from build123d import *

# Parameters (mm, degrees)
SKETCH1_R           = 2.625
BOSS_EXTRUDE1_DEPTH = 6


with BuildPart() as part:
    # Sketch1 → Boss-Extrude1 (new body)
    with BuildSketch(Plane(origin=(0, 0, 0), x_dir=(1, 0, 0), z_dir=(0, 1, 0))):
        with BuildLine():
            Line((-7, 10), (7, 10))
            ThreePointArc((7, 10), (7.707106781, 9.707106781), (8, 9))
            Line((8, 9), (8, -9))
            ThreePointArc((8, -9), (7.707106781, -9.707106781), (7, -10))
            Line((7, -10), (-7, -10))
            ThreePointArc((-7, -10), (-7.707106781, -9.707106781), (-8, -9))
            Line((-8, -9), (-8, 9))
            ThreePointArc((-8, 9), (-7.707106781, 9.707106781), (-7, 10))
        make_face()
        Circle(SKETCH1_R, mode=Mode.SUBTRACT)
    extrude(amount=BOSS_EXTRUDE1_DEPTH)


solid = part.part
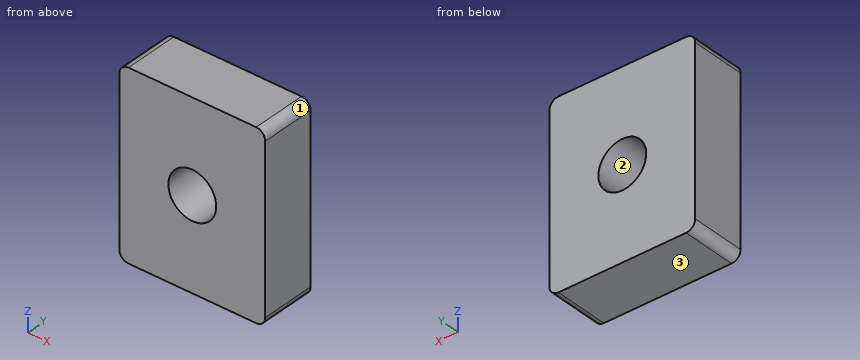
Verification items for the finished model (mm, model axes). Face numbers are marked on the shaded views. Coordinates: 2 decimals unless noted, no trailing zeros. Order: outer loops, then holes, each group sorted by start corner. A loop starts at its lowest first (then second) coordinate and runs counter-clockwise, first axis right, second up. Notation, with made-up numbers: M -15,49.5 L 41,49.5 A16 ccw 41,77.5 Z; hole C 2.25,34 d3. An arc over 180 degrees is marked long. One line per item, written item: value. Start each with the question number.
Item 1: Sectioned sample at C-C on x = 0. Record the cut outline in (y, z) (3 decimals).
Item 2: Thickness scan on probe 1 along X at (y, z) = (4.25, 0) (3 decimals); probe 2 along Z at (x, y) = (0, 3.5) (3 decimals); probe 3 along X at (y, z) = (0.8, 2). Record the ranges inside material, lowest first.
Item 3: Sectioned sample at B-B on y = 3.9. Record the cut outline in (x, z) (3 decimals), then the cut area to 3 significant figures.
Item 4: Sectioned sample at A-A on z = 0. Record the cut outline in (x, y) (3 decimals).
Item 5: Depth check by flat-ended pin: P1, Ø1.5, axis at x = -2.5, z = 2, coming from the -Y side; P2, Ø4.5, axis at x = 0, z = 0, coming from the -Y side. Enter the tip coordinate at first touch or a pass-through.
Item 6: Mould release check, pull along Z, two halves, no side actions. Record for the marked faces 1, 2 and 3: pulls with the +Z half, pulls with the -Z half, needs draft (parallel to the pull), parting line crosses it, or undercut.
Calculated:
1. outline: M 0,-10 L 6,-10 L 6,-2.625 L 0,-2.625 Z; M 0,2.625 L 6,2.625 L 6,10 L 0,10 Z
2. probe 1: -8 to -2.625, 2.625 to 8
2. probe 2: -10 to -2.625, 2.625 to 10
2. probe 3: -8 to -1.7, 1.7 to 8
3. outline: M -8,-9 A1 ccw -7,-10 L 7,-10 A1 ccw 8,-9 L 8,9 A1 ccw 7,10 L -7,10 A1 ccw -8,9 Z; hole C 0,0 d5.25
3. area: 297 mm^2
4. outline: M -8,0 L -2.625,0 L -2.625,6 L -8,6 Z; M 2.625,0 L 8,0 L 8,6 L 2.625,6 Z
5. P1: y = 0
5. P2: through
6. face 1: pulls with the +Z half
6. face 2: undercut
6. face 3: pulls with the -Z half
